The model under review builds one solid part; all positions refer to its coordinate system, in mm. Face numbers are marked on the shaded views. A direction names the side the tool comes from. Round coordinates to 2 decimals unless told otherwise and drop trailing zeros. Write each loop counter-clockwise with the first axis right and the second up, starting at its lowest first coordinate (ties: lowest second). Pieces come first, ordered by that corner, then holes. Notation, with made-up numbers: (36, -7.5) - (52, -7.5) arc R34 cw to (52, 22.5) - close; hole circle Ø5 at (3.25, 63). An arc over 180 degrees is marked (long way). Return JSON: item names as keys, results as strings.
Autodesk Inventor part; units mm, degrees
ref_plane "YZ Plane" through (0, 0, 0) normal (1, 0, 0) x (0, 1, 0)
ref_plane "XZ Plane" through (0, 0, 0) normal (0, 1, 0) x (-1, 0, 0)
ref_plane "XY Plane" through (0, 0, 0) normal (0, 0, 1) x (1, 0, 0)
sketch "Sketch1" plane through (0, 0, 0) normal (0, 1, 0) x (-1, 0, 0)
  circle A0 centre (0, 0) radius 2.8702
  dimension "d0" = 5.7404
extrude "Extrusion1" add sketch "Sketch1" along normal blind 3.4036
sketch "Sketch6" plane through (0, 3.4036, 0) normal (0, 1, 0) x (1, 0, 0)
  circle A0 centre (0, 0) radius 11.938
  dimension "d22" = 23.876
extrude "Extrusion8" add sketch "Sketch6" along normal mid plane 1.9939
sketch "Sketch7" plane through (0, 2.4067, 0) normal (0, -1, 0) x (1, 0, 0)
  circle A0 centre (0, 0) radius 4.445
  circle A1 centre (0, 0) radius 2.8702
  circle A2 centre (0, 0) radius 1.5875
  dimension "d25" = 8.89
  dimension "d26" = 3.175
extrude "Extrusion9" add sketch "Sketch7" along normal up to surface (2.4067 mm away) contours A0
extrude "Extrusion10" cut sketch "Sketch7" along normal through all contours A1 | A2
extrude "Extrusion11" cut sketch "Sketch7" against normal blind 1.9939 contours A2
sketch "Sketch8" plane through (0, 4.4006, 0) normal (0, 1, 0) x (1, 0, 0)
  line L0 (0, 0) -> (-6.2862, 6.2862)
  line L1 (0, 0) -> (8.89, 0) construction
  circle A0 centre (-6.2862, 6.2862) radius 1.5875
  circle A1 centre (-6.2862, -6.2862) radius 1.5875
  circle A2 centre (6.2862, -6.2862) radius 1.5875
  circle A3 centre (6.2862, 6.2862) radius 1.5875
  dimension "d33" = 8.89
  dimension "d34" = 135
  dimension "d35" = 3.175
  dimension "d38" = 360
extrude "Extrusion12" cut sketch "Sketch8" against normal blind 1.9939
properties part number "ServoHornDisc" material "ABS Plastic"
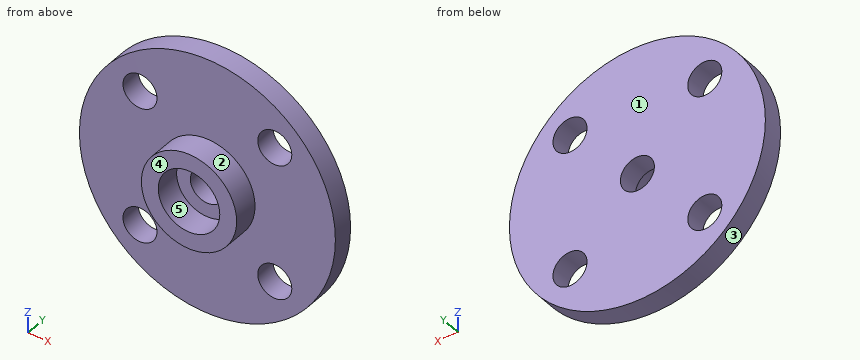
(1) Mouldability with a two-part tool opening along Z and no side actions: class the marked faces 3, 4 and 5 as released by +Z, released by -Z, zero draft, split by the parting line, or undercut.
Filled in:
{"face 3": "split by the parting line", "face 4": "zero draft", "face 5": "undercut"}
(2) Add section C-C (x = 5.25). Write out the cut boundary in (y, z).
Filled in:
{"outline": "(2.41, -10.72) - (4.4, -10.72) - (4.4, -7.49) - (2.41, -7.49) - close; (2.41, -5.08) - (4.4, -5.08) - (4.4, 5.08) - (2.41, 5.08) - close; (2.41, 7.49) - (4.4, 7.49) - (4.4, 10.72) - (2.41, 10.72) - close"}
(3) Add section A-A (x = 0). Write out the cut boundary in (y, z) (1 decimal), plus the area to 3 significant figures.
Filled in:
{"outline": "(0, -4.4) - (2.4, -4.4) - (2.4, -11.9) - (4.4, -11.9) - (4.4, -1.6) - (2.4, -1.6) - (2.4, -2.9) - (0, -2.9) - close; (0, 2.9) - (2.4, 2.9) - (2.4, 1.6) - (4.4, 1.6) - (4.4, 11.9) - (2.4, 11.9) - (2.4, 4.4) - (0, 4.4) - close", "area": "48.9 mm2"}
(4) Add section B-B (z = 0). Write out the cut boundary in (x, y) (1 decimal), plus the area to 3 significant figures.
Filled in:
{"outline": "(-11.9, 2.4) - (-4.4, 2.4) - (-4.4, 0) - (-2.9, 0) - (-2.9, 2.4) - (-1.6, 2.4) - (-1.6, 4.4) - (-11.9, 4.4) - close; (1.6, 2.4) - (2.9, 2.4) - (2.9, 0) - (4.4, 0) - (4.4, 2.4) - (11.9, 2.4) - (11.9, 4.4) - (1.6, 4.4) - close", "area": "48.9 mm2"}
(5) For the marked faces 1 and 2, list the 3-axis set-ups (+Z, -Z, +X, -X, +Y, -Y) from which the entire face can be reached by the end or side of a thin tool; tool diameter is ignored.
Filled in:
{"face 1": "+Z, -Z, +X, -X, +Y", "face 2": "-Y"}
(6) Clearance check with flat-ended pins moving along their axes: pin 1 Ø1.5 at (y, z) = (3, 1.5) entering from +X; pin 2 Ø5 at (x, z) = (6.29, 6.29) entering from -Y; pin 3 Ø2.5 at (x, z) = (-6.29, 6.29) entering from +Y. State where each tip first meets the part, or that it passes through.
Filled in:
{"pin 1": "stops at x = 11.91", "pin 2": "stops at y = 2.41", "pin 3": "passes through"}
(7) Wall thickness on line 1 (Z direction, x = 0, y = 3.2); line 2 (Z direction, x = 6.75, y = 3.8); line 3 (Y direction, x = 9.5, z = -0.75): over which ranges is each line inside the solid? List them lowest first.
Filled in:
{"line 1": "z = -11.94 to -1.59, 1.59 to 11.94", "line 2": "z = -9.85 to -7.8, -4.77 to 4.77, 7.8 to 9.85", "line 3": "y = 2.41 to 4.4"}
(8) Add section D-D (z = -5). Write out the cut boundary in (x, y), plus the area to 3 significant figures.
Filled in:
{"outline": "(-10.84, 2.41) - (-7.22, 2.41) - (-7.22, 4.4) - (-10.84, 4.4) - close; (-5.36, 2.41) - (5.36, 2.41) - (5.36, 4.4) - (-5.36, 4.4) - close; (7.22, 2.41) - (10.84, 2.41) - (10.84, 4.4) - (7.22, 4.4) - close", "area": "35.8 mm2"}
